Design review of the part built by this model. Coordinates are the model's own, in mm. Face numbers are marked on the shaded views. A direction names the side the tool comes from. Round coordinates to 2 decimals unless told otherwise and drop trailing zeros. Write each loop counter-clockwise with the first axis right and the second up, starting at its lowest first coordinate (ties: lowest second). Pieces come first, ordered by that corner, then holes. Notation, with made-up numbers: M 81,19.5 L 107,19.5 A21 ccw 107,48.5 Z; hole C -26.75,-38.75 d9. An arc over 180 degrees is marked long. One line per question, with ' | ' between items. Start each with the question number.
Item 1: For L1, parallel to Z at x = 4, y = 1.5; L2, parallel to X at y = 1.75, z = 5.5; L3, parallel to X at y = 0.75, z = 7.5, list the stretches that pass through material, from the lowest coordinate up.
Item 2: Machinability: for the marked faces 1 and 2, which of the approach directions +Z, -Z, +X, -X, +Y, -Y give a long, thin tool a straight path to every point of the face, cutting with its end or side? Answer none if there is none.
Item 3: Add section C-C, the plane x = 4.25. State the section outline as (y, z) points.
Item 4: Insertion check: pin 1 Ø2 at (y, z) = (4.5, 9) entering from -X; pin 2 Ø1 at (x, z) = (3, 4) entering from -Y; pin 3 Ø2 at (x, z) = (5, 4.5) entering from +Y. Each pin has a flat end and moves straight along its axis. Give the tip position at first contact, or say it passes through.
Item 5: Draft analysis for pull direction Z (two halves, no side actions). For the marked faces 3, 4, 5 and 6, state which applies: released by +Z, released by -Z, zero draft, split by the parting line, or undercut.
Item 6: Add section A-A, the plane z = 8. State the section outline as (x, y) points.
Item 7: Add section D-D, the plane z = 2. State the section outline as (x, y) points.
Item 8: Add section B-B, the plane y = 3.5. State the section outline as (x, z) points, and give its area (3 significant figures).
```python
from build123d import *

# Parameters (mm, degrees)
BOSS_EXTRUDE1_DEPTH = 16
SKETCH4_W           = 4.8
SKETCH4_H           = 12.8
CUT_EXTRUDE2_DEPTH  = 1.8
SHELL1_START        = 1.6
SHELL1_DEPTH        = 12.8
SKETCH2_R           = 1.6
BOSS_EXTRUDE2_DEPTH = 3
SKETCH3_R           = 0.8
CUT_EXTRUDE1_DEPTH  = 3


# Read off the part's stored shape, not the designer's step: Shell1
with BuildPart() as part:
    # Sketch1 → Boss-Extrude1 (new body)
    with BuildSketch(Plane.XY):
        Polygon((0, 0), (0, 2), (8, 6.4), (8, 0), align=None)
    extrude(amount=BOSS_EXTRUDE1_DEPTH)

    # Sketch4 → Cut-Extrude2 (cut)
    with BuildSketch(Plane.XZ):
        with Locations((4, 8)):
            Rectangle(SKETCH4_W, SKETCH4_H)
    extrude(amount=-CUT_EXTRUDE2_DEPTH, mode=Mode.SUBTRACT)

    # Shell1 outline → Shell1 (cut)
    with BuildSketch(Plane.XY.offset(SHELL1_START)):
        Polygon((2.95642537, 1.8), (6.4, 1.8), (6.4, 3.693966046), align=None)
    extrude(amount=SHELL1_DEPTH, mode=Mode.SUBTRACT)

    # Sketch2 → Boss-Extrude2 (add)
    with BuildSketch(Plane.XZ):
        with Locations((4, 8)):
            Circle(SKETCH2_R)
    extrude(amount=-BOSS_EXTRUDE2_DEPTH)

    # Sketch3 → Cut-Extrude1 (cut)
    with BuildSketch(Plane.XZ):
        with Locations((4, 8)):
            Circle(SKETCH3_R)
    extrude(amount=-CUT_EXTRUDE1_DEPTH, mode=Mode.SUBTRACT)


solid = part.part
```
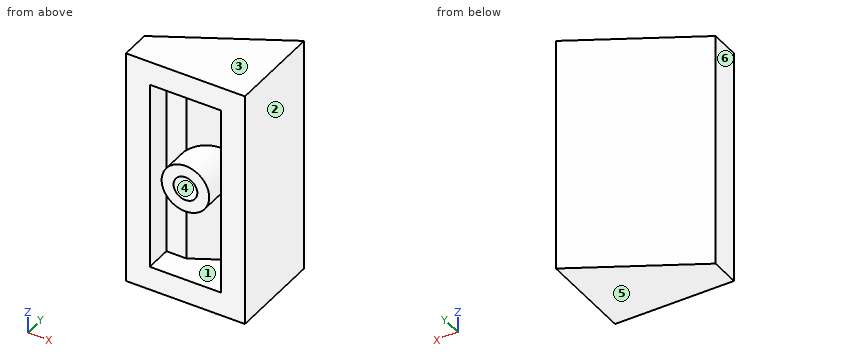
Computed values:
1) L1: z = 0 to 1.6, 6.4 to 7.2, 8.8 to 9.6, 14.4 to 16 | L2: x = 0 to 1.6, 6.4 to 8 | L3: x = 0 to 1.6, 2.48 to 3.38, 4.62 to 5.52, 6.4 to 8
2) face 1: -Y | face 2: +Z, -Z, +X, +Y, -Y
3) outline: M 0,0 L 4.34,0 L 4.34,16 L 0,16 L 0,14.4 L 2.51,14.4 L 2.51,9.58 L 0,9.58 L 0,8.76 L 3,8.76 L 3,7.24 L 0,7.24 L 0,6.42 L 2.51,6.42 L 2.51,1.6 L 0,1.6 Z
4) pin 1: stops at x = 2.73 | pin 2: stops at y = 1.8 | pin 3: stops at y = 5.3
5) face 3: released by +Z | face 4: undercut | face 5: released by -Z | face 6: zero draft
6) outline: M 0,0 L 1.6,0 L 1.6,1.8 L 2.4,1.8 L 2.4,0 L 3.2,0 L 3.2,3 L 4.8,3 L 4.8,0 L 5.6,0 L 5.6,3 L 5.14,3 L 6.4,3.69 L 6.4,0 L 8,0 L 8,6.4 L 0,2 Z
7) outline: M 0,0 L 1.6,0 L 1.6,1.8 L 2.96,1.8 L 6.4,3.69 L 6.4,0 L 8,0 L 8,6.4 L 0,2 Z
8) outline: M 2.73,0 L 8,0 L 8,16 L 2.73,16 Z; hole M 6.05,1.6 L 6.4,1.6 L 6.4,14.4 L 6.05,14.4 Z | area: 79.8 mm^2
